```python
from build123d import *

# Parameters (mm, degrees)
SZKIC1_R                         = 20
DODANIE_WYCI_GNI_CIE1_DEPTH      = 470
DODANIE_WYCI_GNI_CIE2_DEPTH      = 20
DODANIE_WYCI_GNI_CIE2_DEPTH_BACK = 20
WYTNIJ_WYCI_GNI_CIE1_REACH       = 485.115
SZKIC3_R                         = 10
SZKIC4_W                         = 40
SZKIC4_H                         = 40
WYTNIJ_WYCI_GNI_CIE2_DEPTH       = 20
ZAOKR_GLENIE1_R                  = 5
ZAOKR_GLENIE2_R                  = 10


with BuildPart() as part:
    # Szkic1 → Dodanie-wyciągnięcie1 (new body)
    with BuildSketch(Plane(origin=(0, 0, 0), x_dir=(1, 0, 0), z_dir=(0, 1, 0))):
        with Locations(Location((0, 0, 0), (0, 0, 90))):
            Circle(SZKIC1_R)
    extrude(amount=DODANIE_WYCI_GNI_CIE1_DEPTH)

    # Szkic2 → Dodanie-wyciągnięcie2 (add, two sides: drawn at the far end of the back side and taken through both)
    with BuildSketch(Plane.XY.offset(-DODANIE_WYCI_GNI_CIE2_DEPTH_BACK)):
        Polygon((-20, 0), (90, -20), (90, -220), (120, -220), (120, 5.037290602), (-14.633436854, 29.516097303), align=None)
    extrude(amount=DODANIE_WYCI_GNI_CIE2_DEPTH + DODANIE_WYCI_GNI_CIE2_DEPTH_BACK)

    # Szkic3 → Wytnij-wyciągnięcie1 (cut, up to next)
    with BuildSketch(Plane.ZY.offset(-90), mode=Mode.PRIVATE) as wytnij_wyci_gni_cie1_sk1:
        with Locations(Location((0, -200, 0), (0, 0, 270))):
            Circle(SZKIC3_R)
    wytnij_wyci_gni_cie1_tool1 = extrude(wytnij_wyci_gni_cie1_sk1.sketch, amount=-WYTNIJ_WYCI_GNI_CIE1_REACH, mode=Mode.PRIVATE) & part.part
    add(wytnij_wyci_gni_cie1_tool1.solids().sort_by_distance((90, -200, 0))[0], mode=Mode.SUBTRACT)

    # Szkic4 → Wytnij-wyciągnięcie2 (cut)
    with BuildSketch(Plane(origin=(120, 0, 0), x_dir=(0, 0, -1), z_dir=(1, 0, 0))):
        with Locations((0, -200)):
            Rectangle(SZKIC4_W, SZKIC4_H)
    extrude(amount=-WYTNIJ_WYCI_GNI_CIE2_DEPTH, mode=Mode.SUBTRACT)

    # Zaokrąglenie1
    zaokr_glenie1_edges = [part.edges().sort_by_distance(p)[0] for p in [
        (120, -180, 0),
        (100, -180, 0),
    ]]
    fillet(zaokr_glenie1_edges, radius=ZAOKR_GLENIE1_R)

    # Zaokrąglenie2
    zaokr_glenie2_edges = [part.edges().sort_by_distance(p)[0] for p in [
        (95, -220, -20),
        (95, -220, 20),
    ]]
    fillet(zaokr_glenie2_edges, radius=ZAOKR_GLENIE2_R)


solid = part.part
```
Part model, mm, in its own coordinate system. A direction names the side the tool comes from. Round coordinates to 2 decimals unless told otherwise and drop trailing zeros. Loops run counter-clockwise (first coordinate to the right, second up) from the corner with the lowest first, then second, coordinate; pieces in that order, holes last.
Item 1: Mould opens along Z. For faces 1 (the face through (94.93, -209.237, -3.83)), 2 (the face through (91, -54, 20)), 3 (the face through (34.23, -9.86, -0.28)) say: +Z half, -Z half, draft (parallel to the pull), parting line (faces both ways), or undercut.
Item 2: Cut at A-A, the plane y = -200. Give the cut face in (x, z).
Item 3: Cut at D-D, the plane y = 402.5. Give the cut face in (x, z).
Item 4: Cut at B-B, the plane x = 12. Give the cut face in (y, z).
Item 5: 3-axis set-ups, long thin cutter, end or side, ignore diameter. For faces 4 (the face through (-19.83, 231.71, 2.6)), 5 (the face through (90, -119, 0)), 6 (the face through (-17.875, 11.685, 14.304)), 7 (the face through (-17.875, 11.685, -14.584)): which of +Z, -Z, +X, -X, +Y, -Y reach the whole face in a straight line?
Item 6: Cut at C-C, the plane y = -68. Give the cut face in (x, z).
Item 7: Drop flat-ended pins along their axis: P1, Ø4, axis at x = 83, z = -7.5, coming from the -Y side; P2, Ø1, axis at x = 24, z = 12, coming from the +Y side; P3, Ø8, axis at x = 112, z = 9, coming from the -Y side. Give the stop position or say it passes through.
Item 8: Drill centre lines: line 1 (Z direction, x = 98, y = -200); line 2 (Y direction, x = 93, z = 1); line 3 (X direction, y = 211, z = -1). Where is each one in solid material? Low to high.
A:
1. face 1: undercut
1. face 2: +Z half
1. face 3: draft
2. outline: (90, -20) - (100, -20) - (100, -10) - (90, -10) - close; (90, 10) - (100, 10) - (100, 20) - (90, 20) - close
3. outline: circle Ø40 at (0, 0)
4. outline: (-5.82, -20) - (24.67, -20) - (24.67, -16) - (470, -16) - (470, 16) - (24.67, 16) - (24.67, 20) - (-5.82, 20) - close
5. face 4: +Y
5. face 5: +Z, -Z, -X, -Y
5. face 6: +Z, -X, +Y
5. face 7: -Z, -X, +Y
6. outline: (90, -20) - (120, -20) - (120, 20) - (90, 20) - close
7. P1: stops at y = -19.09
7. P2: stops at y = 22.58
7. P3: stops at y = -180
8. line 1: z = -20 to -10, 10 to 20
8. line 2: y = -220 to -209.95, -190.05 to 9.95
8. line 3: x = -19.97 to 19.97
